from build123d import *

# Parameters (mm, degrees)
F0_R     = 40.072412
F0_R_2   = 34.84556
F1_DEPTH = 25.4
F0_R_3   = 17.387916
F2_DEPTH = 50.8
F0_R_4   = 8.335342
F3_DEPTH = 101.6
F4_DEPTH = 127


with BuildPart() as f1:
    # F0 (on Front) → F1 (new body)
    with BuildSketch(Plane.XZ):
        Circle(F0_R)
        Circle(F0_R_2, mode=Mode.SUBTRACT)
    extrude(amount=F1_DEPTH)

    # F0 (on Front) → F2 (join)
    with BuildSketch(Plane.XZ):
        Circle(F0_R_2)
        Circle(F0_R_3, mode=Mode.SUBTRACT)
    extrude(amount=F2_DEPTH)

    # F0 (on Front) → F3 (join)
    with BuildSketch(Plane.XZ):
        Circle(F0_R_3)
        Circle(F0_R_4, mode=Mode.SUBTRACT)
    extrude(amount=F3_DEPTH)

    # F0 (on Front) → F4 (join)
    with BuildSketch(Plane.XZ):
        Circle(F0_R_4)
    extrude(amount=F4_DEPTH)


solid = f1.part
Design review of the part built by this model. Coordinates are the model's own, in mm. A direction names the side the tool comes from. Coordinates: 2 decimals unless noted, no trailing zeros. Loops run counter-clockwise (first coordinate to the right, second up) from the corner with the lowest first, then second, coordinate; pieces in that order, holes last. Notation, with made-up numbers: (63, 12.25) -> (97, 12.25) arc R18 cw to (97, 36.25) -> close; hole circle Ø1 at (1, -27). An arc over 180 degrees is marked (long way). Use a Markdown table: item, result. Add a question column.
Item 1: We need section A-A, the plane z = 0. Write out the cut boundary in (x, y).
Item 2: Clearance check with flat-ended pins moving along their axes: P1, Ø2, axis at x = -10.5, y = -93.5, coming from the -Z side; P2, Ø10, axis at y = -60.5, z = 3, coming from the -X side; P3, Ø12, axis at x = -5, z = -26.5, coming from the -Y side. State where each tip first meets the part, or that it passes through.
Item 3: We need section C-C, the plane y = -16. Write out the cut boundary in (x, z).
Item 4: Wall thickness on L1, parallel to Y at x = -7, z = -12; L2, parallel to Y at x = 28.5, z = -7.5; L3, parallel to Z at x = -1, y = -39: over which ranges is each line inside the solid? List them lowest first. Write a range as from..to.
Item 5: We need section B-B, the plane x = 0. Write out the cut boundary in (y, z).
Item 6: Machinability: for faces 1 (the flat face through (7.5, -101.6, 4.1)), 2 (the flat face through (0, -127, 0)), which of the approach directions +Z, -Z, +X, -X, +Y, -Y give a long, thin tool a straight path to every point of the face, cutting with its end or side? Answer none if there is none.
Item 7: We need section D-D, the plane x = -24. Write out the cut boundary in (y, z).
Numbers:
| question | item | result |
|---|---|---|
| 1 | outline | (-40.07, -25.4) -> (-34.85, -25.4) -> (-34.85, -50.8) -> (-17.39, -50.8) -> (-17.39, -101.6) -> (-8.34, -101.6) -> (-8.34, -127) -> (8.34, -127) -> (8.34, -101.6) -> (17.39, -101.6) -> (17.39, -50.8) -> (34.85, -50.8) -> (34.85, -25.4) -> (40.07, -25.4) -> (40.07, 0) -> (-40.07, 0) -> close |
| 2 | P1 | stops at z = -14.56 |
| 2 | P2 | stops at x = -17.39 |
| 2 | P3 | stops at y = -50.8 |
| 3 | outline | circle Ø80.14 at (0, 0) |
| 4 | L1 | y = -101.6..0 |
| 4 | L2 | y = -50.8..0 |
| 4 | L3 | z = -34.83..34.83 |
| 5 | outline | (-127, -8.34) -> (-101.6, -8.34) -> (-101.6, -17.39) -> (-50.8, -17.39) -> (-50.8, -34.85) -> (-25.4, -34.85) -> (-25.4, -40.07) -> (0, -40.07) -> (0, 40.07) -> (-25.4, 40.07) -> (-25.4, 34.85) -> (-50.8, 34.85) -> (-50.8, 17.39) -> (-101.6, 17.39) -> (-101.6, 8.34) -> (-127, 8.34) -> close |
| 6 | face 1 | -Y |
| 6 | face 2 | +Z, -Z, +X, -X, -Y |
| 7 | outline | (-50.8, -25.26) -> (-25.4, -25.26) -> (-25.4, -32.09) -> (0, -32.09) -> (0, 32.09) -> (-25.4, 32.09) -> (-25.4, 25.26) -> (-50.8, 25.26) -> close |
